Read the model definition and answer for the solid it produces. Units are mm, in the model's axes. Face numbers are marked on the shaded views. A direction names the side the tool comes from. Coordinates: 2 decimals unless noted, no trailing zeros. Write each loop counter-clockwise with the first axis right and the second up, starting at its lowest first coordinate (ties: lowest second). Pieces come first, ordered by that corner, then holes. Notation, with made-up numbers: M -12,11 L 21,11 A23 cw 21,25 Z; hole C 46,-24.75 d5. An arc over 180 degrees is marked long. Use a Markdown table: item, result. Add a question column.
from build123d import *

# Parameters (mm, degrees)
ESBO_O1_R                = 10
RESSALTO_EXTRUS_O1_DEPTH = 3
ESBO_O2_R                = 6
RESSALTO_EXTRUS_O2_DEPTH = 12
ESBO_O3_R                = 4.05
CORTE_EXTRUS_O1_DEPTH    = 21.615528128


with BuildPart() as part:
    # Esboço1 → Ressalto-extrusão1 (new body)
    with BuildSketch(Plane(origin=(0, 0, 0), x_dir=(1, 0, 0), z_dir=(0, 1, 0))):
        with Locations(Location((0, 0, 0), (0, 0, 270))):
            Circle(ESBO_O1_R)
    extrude(amount=RESSALTO_EXTRUS_O1_DEPTH)

    # Esboço2 → Ressalto-extrusão2 (add)
    with BuildSketch(Plane(origin=(0, 3, 0), x_dir=(1, 0, 0), z_dir=(0, 1, 0))):
        with Locations(Location((0, 0, 0), (0, 0, 270))):
            Circle(ESBO_O2_R)
    extrude(amount=RESSALTO_EXTRUS_O2_DEPTH)

    # Esboço3 → Corte-extrusão1 (cut, through all)
    with BuildSketch(Plane(origin=(0, 15, 0), x_dir=(1, 0, 0), z_dir=(0, 1, 0))):
        with Locations(Location((0, 0, 0), (0, 0, 270))):
            Circle(ESBO_O3_R)
    extrude(amount=-CORTE_EXTRUS_O1_DEPTH, mode=Mode.SUBTRACT)


solid = part.part
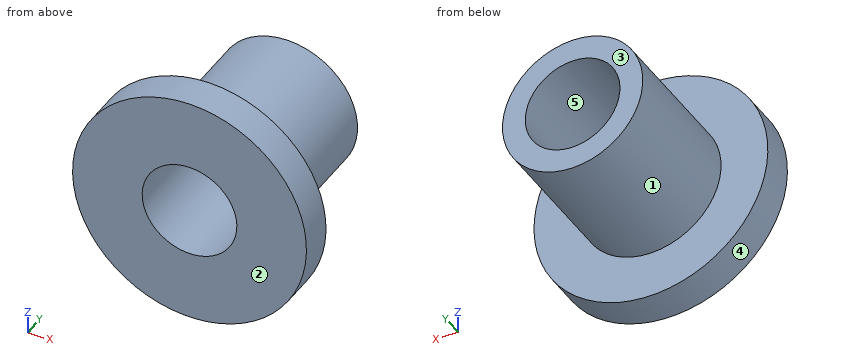
Item 1: Each of these flat-tipped pins is pushed along its axis until it touches: pin 1 (1 mm diameter, centred on y = 2, z = 2.5, fed in from -X); pin 2 (2 mm diameter, centred on x = 0.5, y = 11, fed in from -Z); pin 3 (3 mm diameter, centred on x = 2.5, y = 2, fed in from +Z); pin 4 (6.5 mm diameter, centred on x = 0, z = 0, fed in from +Y) (3 decimals). Where does it stop, or does it pass through?
Item 2: Find section B-B on x = 0. Give the vertices of the cut face in (y, z), then the cut area to 3 significant figures.
Item 3: Find section D-D on x = 7.5. Give the vertices of the cut face in (y, z).
Item 4: For the marked faces 1 and 2, determine the directions among +Z, -Z, +X, -X, +Y, -Y from which every point of the face is accessible in a straight line to the end or side of a thin tool.
Item 5: Find section A-A on z = 0. Give the vertices of the cut face in (x, y), then the cut area to 3 significant figures.
Item 6: Find section C-C on y = 10.5. Give the vertices of the cut face in (x, z).
Item 7: Determine the mould class of the marked faces 3, 4 and 5 for opening direction X: pulls with the +X half, pulls with the -X half, needs draft (parallel to the pull), parting line crosses it, or undercut.
Item 8: Consider probe 1 along X at (y, z) = (4.25, 0); probe 2 along Y at (x, z) = (2.25, 5.75); probe 3 along Z at (x, y) = (-9, 0.5). Determine where each line is inside the solid, lowest interval first.
Geometry says:
| question | item | result |
|---|---|---|
| 1 | pin 1 | stops at x = -9.8 |
| 1 | pin 2 | stops at z = -6 |
| 1 | pin 3 | stops at z = 9.95 |
| 1 | pin 4 | passes through |
| 2 | outline | M 0,-10 L 3,-10 L 3,-6 L 15,-6 L 15,-4.05 L 0,-4.05 Z; M 0,4.05 L 15,4.05 L 15,6 L 3,6 L 3,10 L 0,10 Z |
| 2 | area | 82.5 mm2 |
| 3 | outline | M 0,-6.61 L 3,-6.61 L 3,6.61 L 0,6.61 Z |
| 4 | face 1 | +Y |
| 4 | face 2 | +Z, -Z, +X, -X, -Y |
| 5 | outline | M -10,0 L -4.05,0 L -4.05,15 L -6,15 L -6,3 L -10,3 Z; M 4.05,0 L 10,0 L 10,3 L 6,3 L 6,15 L 4.05,15 Z |
| 5 | area | 82.5 mm2 |
| 6 | outline | C 0,0 d12; hole C 0,0 d8.1 |
| 7 | face 3 | needs draft |
| 7 | face 4 | parting line crosses it |
| 7 | face 5 | undercut |
| 8 | probe 1 | x = -6 to -4.05, 4.05 to 6 |
| 8 | probe 2 | y = 0 to 3 |
| 8 | probe 3 | z = -4.36 to 4.36 |
